Input: dimensioned drawing with shaded views. Units: mm. Origin: part minimum x, y, z. Give positions to 0.01 mm unless a question says otherwise; leave off trailing zeros. Loops run counter-clockwise (first coordinate to the right, second up) from the corner with the lowest first, then second, coordinate; pieces in that order, holes last. Notation, with made-up numbers: (83, 63) -> (99, 63) arc R23 ccw to (99, 84) -> close; hole circle Ø1 at (-10, 62.5). An arc over 180 degrees is marked (long way). One line per question, with ' | ' between items. Start each with the question number.
Item 1: Section C-C on z = 12.7. Give the number of separate pieces and of enclosed holes in the cut face, then the cut area to 3 significant figures.
Item 2: Section B-B on x = 19.05. Return loops of the section in (y, z) (1 decimal), then the cut area to 3 significant figures.
Item 3: Material intervals for line 1 along X through (y, z) = (1.6, 76.2); line 2 along Z through (x, y) = (19.05, 2.4); line 3 along Z through (x, y) = (14, 2.9), sorted ascending. Write a range as [from, to].
Item 4: Pin query (flat end, axial travel): P1, Ø1, axis at x = 20, y = 2, coming from the +Z side. Return the tip coordinate at first contact, or that it passes through.
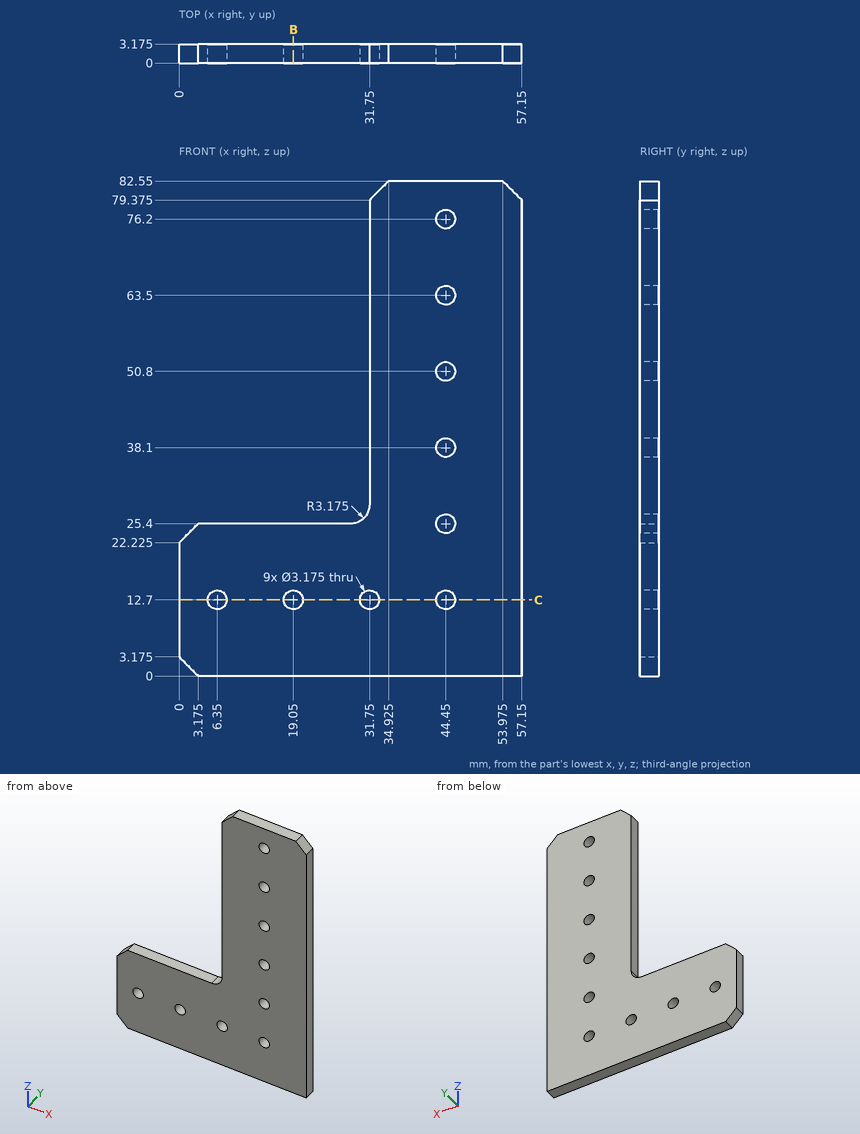
Result sheet:
1) separate pieces: 5 | enclosed holes: 0 | area: 141 mm²
2) outline: (0, 0) -> (3.2, 0) -> (3.2, 11.1) -> (0, 11.1) -> close; (0, 14.3) -> (3.2, 14.3) -> (3.2, 25.4) -> (0, 25.4) -> close | area: 70.6 mm²
3) line 1: x = [31.75, 42.86], [46.04, 57.15] | line 2: z = [0, 11.11], [14.29, 25.4] | line 3: z = [0, 25.4]
4) P1: stops at z = 25.4
